Check sheet for the modelled part. Datum: model origin and axes. Units: mm. Face numbers are marked on the shaded views. A direction names the side the tool comes from. Round coordinates to 2 decimals unless told otherwise and drop trailing zeros. Order: outer loops, then holes, each group sorted by start corner. A loop starts at its lowest first (then second) coordinate and runs counter-clockwise, first axis right, second up. Notation, with made-up numbers: (55.25, 85) -> (93.25, 85) arc R15 ccw to (93.25, 108) -> close; hole circle Ø9 at (36, 66). An arc over 180 degrees is marked (long way). Answer in a Markdown table with one row per item.
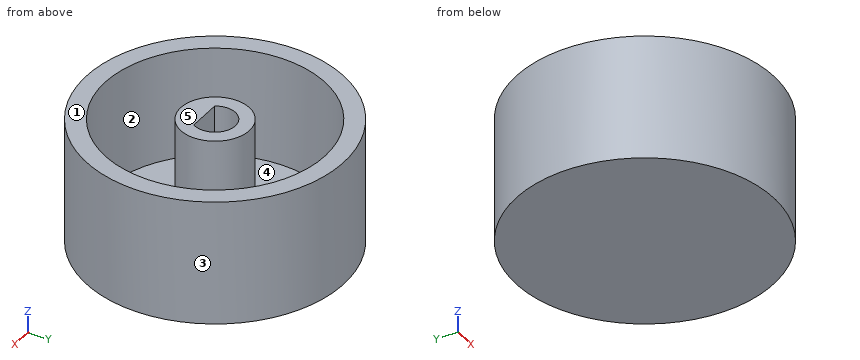
from build123d import *

# Parameters (mm, degrees)
F0_R     = 10.4775
F1_DEPTH = 1.27
F2_R     = 10.4775
F2_R_2   = 8.9535
F2_R_3   = 2.794
F3_DEPTH = 8.89


# Not quite as in the source:
# - the program builds the solid bodies; features that only make, move or delete a surface that nothing else refers to are left out


with BuildPart() as f1:
    # F0 (on Top) → F1 (new body)
    with BuildSketch(Plane.XY):
        Circle(F0_R)
    extrude(amount=F1_DEPTH)

    # F2 (on face) → F3 (join)
    with BuildSketch(Plane.XY.offset(1.27)):
        Circle(F2_R)
        Circle(F2_R_2, mode=Mode.SUBTRACT)
        Circle(F2_R_3)
        with BuildLine():
            ThreePointArc((-1.397, -0.8798818102), (0, 1.651), (1.397, -0.8798818102))
            Line((1.397, -0.8798818102), (-1.397, -0.8798818102))
        make_face(mode=Mode.SUBTRACT)
    extrude(amount=F3_DEPTH)


solid = f1.part
Item 1: Cross-section at C-C (x = 0). Record the boundary of the cut face in (y, z), and give its area (3 significant figures).
Result sheet:
| item | result |
|---|---|
| outline | (-10.48, 0) -> (10.48, 0) -> (10.48, 10.16) -> (8.95, 10.16) -> (8.95, 1.27) -> (2.79, 1.27) -> (2.79, 10.16) -> (1.65, 10.16) -> (1.65, 1.27) -> (-0.88, 1.27) -> (-0.88, 10.16) -> (-2.79, 10.16) -> (-2.79, 1.27) -> (-8.95, 1.27) -> (-8.95, 10.16) -> (-10.48, 10.16) -> close |
| area | 80.9 mm^2 |
Item 2: Set-up check for the marked faces 1 and 2: record each of +Z, -Z, +X, -X, +Y, -Y from which the full face is reachable in a straight line by a thin tool's end or side.
Result sheet:
| item | result |
|---|---|
| face 1 | +Z, +X, -X, +Y, -Y |
| face 2 | +Z |
Item 3: Mould release check, pull along X, two halves, no side actions. Record for the marked faces 3, 4 and 5: pulls with the +X half, pulls with the -X half, needs draft (parallel to the pull), parting line crosses it, or undercut.
Result sheet:
| item | result |
|---|---|
| face 3 | parting line crosses it |
| face 4 | undercut |
| face 5 | needs draft |
Item 4: Depth check by flat-ended pin: P1, Ø2, axis at x = -5.5, z = 6.5, coming from the -Y side; P2, Ø5, axis at x = -4.5, z = 8.5, coming from the -Y side; P3, Ø1, axis at x = -4.5, z = 4.5, coming from the -Y side. Enter the tip coordinate at first touch or a pass-through.
Result sheet:
| item | result |
|---|---|
| P1 | stops at y = -9.46 |
| P2 | stops at y = -10.28 |
| P3 | stops at y = -9.68 |
Item 5: Cross-section at D-D (x = -4). Record the boundary of the cut face in (y, z), and give its area (3 significant figures).
Result sheet:
| item | result |
|---|---|
| outline | (-9.68, 0) -> (9.68, 0) -> (9.68, 10.16) -> (8.01, 10.16) -> (8.01, 1.27) -> (-8.01, 1.27) -> (-8.01, 10.16) -> (-9.68, 10.16) -> close |
| area | 54.4 mm^2 |
Item 6: Scan lines: line 1 (Y direction, x = 0, z = 8.25); line 2 (X direction, y = 2.5, z = 4.5); line 3 (X direction, y = -0.5, z = 9.25). Record each from-to range of solid material in increasing order. Write a range as [from, to].
Result sheet:
| item | result |
|---|---|
| line 1 | y = [-10.48, -8.95], [-2.79, -0.88], [1.65, 2.79], [8.95, 10.48] |
| line 2 | x = [-10.17, -8.6], [-1.25, 1.25], [8.6, 10.17] |
| line 3 | x = [-10.47, -8.94], [-2.75, -1.57], [1.57, 2.75], [8.94, 10.47] |
Item 7: Cross-section at B-B (y = 0). Record the boundary of the cut face in (x, z).
Result sheet:
| item | result |
|---|---|
| outline | (-10.48, 0) -> (10.48, 0) -> (10.48, 10.16) -> (8.95, 10.16) -> (8.95, 1.27) -> (2.79, 1.27) -> (2.79, 10.16) -> (1.65, 10.16) -> (1.65, 1.27) -> (-1.65, 1.27) -> (-1.65, 10.16) -> (-2.79, 10.16) -> (-2.79, 1.27) -> (-8.95, 1.27) -> (-8.95, 10.16) -> (-10.48, 10.16) -> close |
Item 8: Cross-section at A-A (z = 6). Record the boundary of the cut face in (x, y) (1 decimal).
Result sheet:
| item | result |
|---|---|
| outline | circle Ø21 at (0, 0); circle Ø5.6 at (0, 0); hole circle Ø17.9 at (0, 0); hole (-1.4, -0.9) -> (1.4, -0.9) arc R1.7 ccw (long way) to start |
